Part model, mm, in its own coordinate system. Face numbers are marked on the shaded views. A direction names the side the tool comes from. Coordinates: 2 decimals unless noted, no trailing zeros. Loops run counter-clockwise (first coordinate to the right, second up) from the corner with the lowest first, then second, coordinate; pieces in that order, holes last. Notation, with made-up numbers: (0, -39.5) -> (26, -39.5) arc R19 ccw to (26, -24.5) -> close; hole circle Ø3 at (-8.75, -27). An arc over 180 degrees is marked (long way). One line per question, with ' | ' between items. Start each with the question number.
1) Cut at B-B (z = 2.25). List the corners of the cut face in (x, y), plus the area to 3 significant figures.
2) 3-axis set-ups, long thin cutter, end or side, ignore diameter. For the marked faces 1 and 2: which of +Z, -Z, +X, -X, +Y, -Y reach the whole face in a straight line?
3) Cut at D-D (z = 23.25). List the corners of the cut face in (x, y).
4) Drop flat-ended pins along their axis: pin 1 (12 mm diameter, centred on x = -16.5, y = 43, fed in from +Z); pin 2 (1.2 mm diameter, centred on x = 36, z = 1, fed in from +Y); pin 3 (4 mm diameter, centred on y = 11, z = 20.5, fed in from +X). Give the stop position or say it passes through.
5) Two-plate mould, pull along Y, no slides. Class the marked faces 3, 4, 5 and 6: released by +Y, released by -Y, zero draft, split by the parting line, or undercut.
6) Probe L1, parallel to Y at x = -4.5, z = 13.5; L2, parallel to X at y = 24.5, z = 23; L3, parallel to Z at x = 23, y = 49. List the from-to ranges inside material, lowest first. Write a range as from..to.
7) Cut at C-C (x = -26). List the corners of the cut face in (y, z), plus the area to 3 significant figures.
8) Cut at A-A (y = 39). List the corners of the cut face in (x, z).
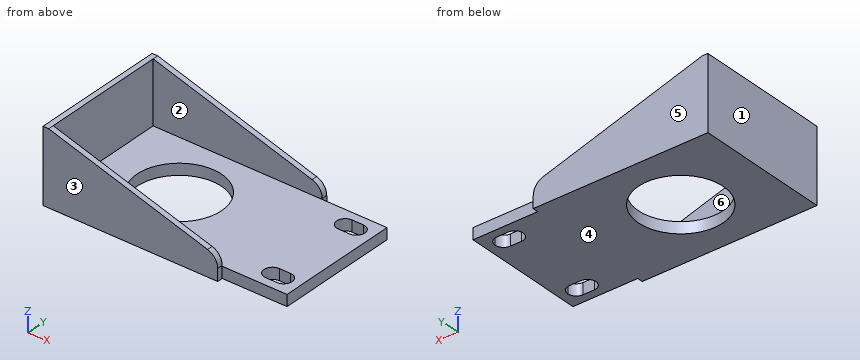
from build123d import *

# Parameters (mm, degrees)
F0_W      = 77
F0_H      = 44
F0_R      = 15
F1_DEPTH  = 4
F2_W      = 54
F2_H      = 2
F3_DEPTH  = 4
F4_W      = 2
F4_H      = 48
F5_DEPTH  = 4
F6_W      = 2
F6_H      = 48
F7_DEPTH  = 22
F9_DEPTH  = 2
F11_DEPTH = 2
F12_R     = 5
F13_R     = 5


with BuildPart() as f1:
    # F0 (on Top) → F1 (new body)
    with BuildSketch(Plane.XY):
        with Locations((5.464885, 29.412094)):
            Rectangle(F0_W, F0_H)
        with BuildLine():
            ThreePointArc((37.964885, 16.412094), (40.086206, 15.533415), (40.964885, 13.412094))
            ThreePointArc((40.964885, 13.412094), (40.086206, 11.290774), (37.964885, 10.412094))
            Line((37.964885, 10.412094), (33.964885, 10.412094))
            ThreePointArc((33.964885, 10.412094), (30.964885, 13.412094), (33.964885, 16.412094))
            Line((33.964885, 16.412094), (37.964885, 16.412094))
        make_face(mode=Mode.SUBTRACT)
        with Locations((-12.035115, 29.412094)):
            Circle(F0_R, mode=Mode.SUBTRACT)
        with BuildLine():
            ThreePointArc((37.964885, 48.412094), (40.086206, 47.533415), (40.964885, 45.412094))
            ThreePointArc((40.964885, 45.412094), (40.086206, 43.290774), (37.964885, 42.412094))
            Line((37.964885, 42.412094), (33.964885, 42.412094))
            ThreePointArc((33.964885, 42.412094), (30.964885, 45.412094), (33.964885, 48.412094))
            Line((33.964885, 48.412094), (37.964885, 48.412094))
        make_face(mode=Mode.SUBTRACT)
    extrude(amount=F1_DEPTH)



with BuildPart() as f3:
    # F2 (on face) → F3 (new body)
    with BuildSketch(Plane.XY.offset(4)):
        with Locations((-6.035115, 52.412094)):
            Rectangle(F2_W, F2_H)
        Polygon((-33.035115, 7.412094), (-33.035115, 51.412094), (-33.035115, 53.412094), (-39.035115, 53.412094), (-39.035115, 5.412094), (-33.035115, 5.412094), align=None)
        with Locations((-6.035115, 6.412094)):
            Rectangle(F2_W, F2_H)
    extrude(amount=-F3_DEPTH)

    # F4 (on face) → F5 (join)
    with BuildSketch(Plane.XY.offset(4)):
        with Locations((-40.035115, 29.412094)):
            Rectangle(F4_W, F4_H)
    extrude(amount=-F5_DEPTH)

    # F6 (on face) → F7 (join)
    with BuildSketch(Plane.XY.offset(4)):
        with Locations((-40.035115, 29.412094)):
            Rectangle(F6_W, F6_H)
    extrude(amount=F7_DEPTH)


with BuildPart() as f1_1:
    add(f1.part)

    add(f3.part)  # F9 merges F3
    # F8 (on face) → F9 (join)
    with BuildSketch(Plane.XZ.offset(-5.412094)):
        Polygon((-39.035115, 4), (20.964885, 4), (20.964885, 8), (-39.035115, 26), align=None)
    extrude(amount=-F9_DEPTH)

    # F10 (on face) → F11 (join)
    with BuildSketch(Plane(origin=(0, 53.412094, 0), x_dir=(-1, 0, 0), z_dir=(0, 1, 0))):
        Polygon((-20.964885, 8), (-20.964885, 4), (39.035115, 4), (39.035115, 26), align=None)
    extrude(amount=-F11_DEPTH)

    # F12
    f12_edges = [f1_1.edges().sort_by_distance(p)[0] for p in [
        (20.964885, 52.412094, 8),
    ]]
    fillet(f12_edges, radius=F12_R)

    # F13
    f13_edges = [f1_1.edges().sort_by_distance(p)[0] for p in [
        (20.964885, 6.412094, 8),
    ]]
    fillet(f13_edges, radius=F13_R)


solid = f1_1.part
Reported:
1) outline: (-41.04, 5.41) -> (20.96, 5.41) -> (20.96, 7.41) -> (43.96, 7.41) -> (43.96, 51.41) -> (20.96, 51.41) -> (20.96, 53.41) -> (-41.04, 53.41) -> close; hole circle Ø30 at (-12.04, 29.41); hole (33.96, 10.41) -> (37.96, 10.41) arc R3 ccw to (40.96, 13.41) arc R3 ccw to (37.96, 16.41) -> (33.96, 16.41) arc R3 ccw to start; hole (33.96, 42.41) -> (37.96, 42.41) arc R3 ccw to (40.96, 45.41) arc R3 ccw to (37.96, 48.41) -> (33.96, 48.41) arc R3 ccw to start | area: 3,180 mm²
2) face 1: +Z, -Z, -X, +Y, -Y | face 2: +Z, +X
3) outline: (-41.04, 5.41) -> (-29.87, 5.41) -> (-29.87, 7.41) -> (-39.04, 7.41) -> (-39.04, 51.41) -> (-29.87, 51.41) -> (-29.87, 53.41) -> (-41.04, 53.41) -> close
4) pin 1: stops at z = 4 | pin 2: stops at y = 51.41 | pin 3: stops at x = -39.04
5) face 3: released by -Y | face 4: zero draft | face 5: released by +Y | face 6: undercut
6) L1: y = 5.41..7.41, 51.41..53.41 | L2: x = -41.04..-39.04 | L3: z = 0..4
7) outline: (5.41, 0) -> (23.94, 0) -> (23.94, 4) -> (7.41, 4) -> (7.41, 22.09) -> (5.41, 22.09) -> close; (34.89, 0) -> (53.41, 0) -> (53.41, 22.09) -> (51.41, 22.09) -> (51.41, 4) -> (34.89, 4) -> close | area: 221 mm²
8) outline: (-41.04, 0) -> (-23.57, 0) -> (-23.57, 4) -> (-39.04, 4) -> (-39.04, 26) -> (-41.04, 26) -> close; (-0.5, 0) -> (43.96, 0) -> (43.96, 4) -> (-0.5, 4) -> close
